Part model, mm, in its own coordinate system. A direction names the side the tool comes from. Give positions to 0.01 mm unless a question says otherwise; leave off trailing zeros. Write each loop counter-clockwise with the first axis right and the second up, starting at its lowest first coordinate (ties: lowest second). Pieces come first, ordered by that corner, then holes. Notation, with made-up numbers: M -35.75,10.25 L 0.25,10.25 A13 ccw 0.25,14.25 Z; hole C 84,-36 d10. An arc over 180 degrees is marked long. Use CSV: the item, a comma, the result in double quotes. Start each with the question number.
Item 1: Pin check, flat tips, straight feed: pin 1 (1.5 mm diameter, centred on x = 1.5, y = 2.5, fed in from +Z); pin 2 (1.2 mm diameter, centred on x = 0.5, z = -1.5, fed in from -Y). Stop position of each tip, or through.
Item 2: Cut at A-A (y = 1.6). List the corners of the cut face in (x, z), then the cut area to 3 significant figures.
Item 3: Cut at D-D (z = -1.85). List the corners of the cut face in (x, y).
Item 4: Cut at C-C (y = 4.1). List the corners of the cut face in (x, z), then the cut area to 4 significant figures.
Item 5: Mould opens along X. For faces 4 (the flat face through (0, 3, 0)), 5 (the flat face through (0, 5, -1)), 6 (the flat face through (17.5, 2, 0)), 7 (the flat face through (-17.5, 2, 0)) say: released by +X, released by -X, zero draft, split by the parting line, or undercut.
Item 6: Drill centre lines: line 1 (X direction, y = 0.6, z = 1.5); line 2 (X direction, y = 1.65, z = -1.6); line 3 (Z direction, x = -4.5, y = 0.4). Where is each one in solid material? Low to high. Write a range as [from, to].
Item 7: Which spindle directions (+Z, -Z, +X, -X, +Y, -Y) get a long thin tool onto all of the face, cutting with end or side? Do faces 1 (the flat face through (7.5, 2, 1)), 2 (the flat face through (-12, 0, 0)), 3 (the flat face through (2.5, 1, -1)). Say none if no direction does.
Item 8: Cut at B-B (z = 0.4). List the corners of the cut face in (x, y), then the cut area to 3 significant figures.
from build123d import *

# Parameters (mm, degrees)
F0_W     = 17.5
F0_H     = 5
F1_DEPTH = 2.5
F2_W     = 7.5
F2_H     = 5
F3_DEPTH = 2.5
F4_W     = 2.5
F4_H     = 2.5
F5_DEPTH = 2.5


with BuildPart() as f1:
    # F0 (on Top) → F1 (new body, symmetric)
    with BuildSketch(Plane.XY):
        with Locations((8.75, 2.5)):
            Rectangle(F0_W, F0_H)
        with Locations((-8.75, 2.5)):
            Rectangle(F0_W, F0_H)
    extrude(amount=F1_DEPTH, both=True)

    # F2 (on Top) → F3 (cut)
    with BuildSketch(Plane.XY):
        with Locations((3.75, 2.5)):
            Rectangle(F2_W, F2_H)
        with Locations((-3.75, 2.5)):
            Rectangle(F2_W, F2_H)
    extrude(amount=F3_DEPTH, mode=Mode.SUBTRACT)

    # F4 (on Right) → F5 (cut, symmetric)
    with BuildSketch(Plane.YZ):
        with Locations((1.25, -1.25)):
            Rectangle(F4_W, F4_H)
    extrude(amount=F5_DEPTH, both=True, mode=Mode.SUBTRACT)


solid = f1.part
Worked answers:
1,pin 1,"stops at z = 0"
1,pin 2,"stops at y = 2.5"
2,outline,"M -17.5,-2.5 L -2.5,-2.5 L -2.5,0 L -7.5,0 L -7.5,2.5 L -17.5,2.5 Z; M 2.5,-2.5 L 17.5,-2.5 L 17.5,2.5 L 7.5,2.5 L 7.5,0 L 2.5,0 Z"
2,area,"125 mm^2"
3,outline,"M -17.5,0 L -2.5,0 L -2.5,2.5 L 2.5,2.5 L 2.5,0 L 17.5,0 L 17.5,5 L -17.5,5 Z"
4,outline,"M -17.5,-2.5 L 17.5,-2.5 L 17.5,2.5 L 7.5,2.5 L 7.5,0 L -7.5,0 L -7.5,2.5 L -17.5,2.5 Z"
4,area,"137.5 mm^2"
5,face 4,"undercut"
5,face 5,"zero draft"
5,face 6,"released by +X"
5,face 7,"released by -X"
6,line 1,"x = [-17.5, -7.5], [7.5, 17.5]"
6,line 2,"x = [-17.5, -2.5], [2.5, 17.5]"
6,line 3,"z = [-2.5, 0]"
7,face 1,"+Z, +Y, -Y"
7,face 2,"+Z, -Z, +X, -X, -Y"
7,face 3,"+Z, -Z, -Y"
8,outline,"M -17.5,0 L -7.5,0 L -7.5,5 L -17.5,5 Z; M 7.5,0 L 17.5,0 L 17.5,5 L 7.5,5 Z"
8,area,"100 mm^2"
